Verification items for the finished model (mm, model axes). Coordinates: 2 decimals unless noted, no trailing zeros. Write each loop counter-clockwise with the first axis right and the second up, starting at its lowest first coordinate (ties: lowest second). Pieces come first, ordered by that corner, then holes. Notation, with made-up numbers: (33.5, -23.75) -> (60.5, -23.75) arc R11 ccw to (60.5, -5.75) -> close; hole circle Ø5 at (22.25, 17). An arc over 180 degrees is marked (long way). Answer in a Markdown table with one row per item.
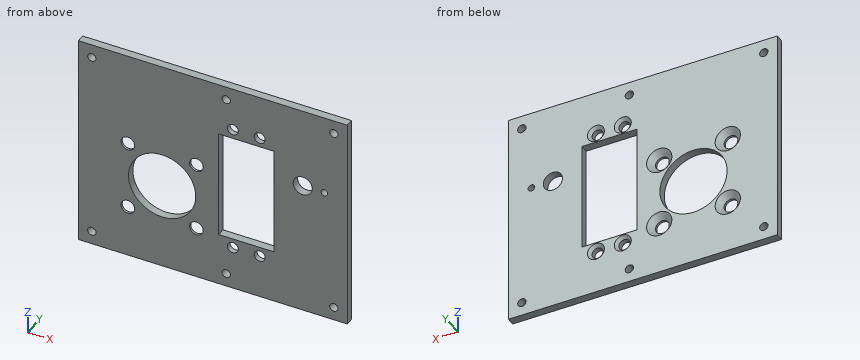
```python
from build123d import *

# Parameters (mm, degrees)
SZKIC1_W                                     = 100
SZKIC1_H                                     = 80
SZKIC1_R                                     = 12.5
SZKIC1_R_2                                   = 2.55
SZKIC1_R_3                                   = 2.05
SZKIC1_R_4                                   = 3.55
SZKIC1_R_5                                   = 1.55
SZKIC1_R_6                                   = 1.25
SZKIC1_W_2                                   = 20.5
SZKIC1_H_2                                   = 40.5
DODANIE_WYCI_GNI_CIE1_DEPTH                  = 3
CSK_FOR_M4_COUNTERSUNK_FLAT_HEAD_SCR_2_COUNT = 2
CSK_FOR_M4_COUNTERSUNK_FLAT_HEAD_SCR_2_PITCH = 25.5
CSK_FOR_M4_COUNTERSUNK_FLAT_HEAD_SCR_3_COUNT = 2
CSK_FOR_M4_COUNTERSUNK_FLAT_HEAD_SCR_3_PITCH = 36.062445841
CSK_FOR_M4_COUNTERSUNK_FLAT_HEAD_SCR_4_COUNT = 2
CSK_FOR_M4_COUNTERSUNK_FLAT_HEAD_SCR_4_PITCH = 25.5
CSK_FOR_M3_COUNTERSUNK_FLAT_HEAD_SCR_2_COUNT = 2
CSK_FOR_M3_COUNTERSUNK_FLAT_HEAD_SCR_2_PITCH = 10
CSK_FOR_M3_COUNTERSUNK_FLAT_HEAD_SCR_3_COUNT = 2
CSK_FOR_M3_COUNTERSUNK_FLAT_HEAD_SCR_3_PITCH = 47.5
CSK_FOR_M3_COUNTERSUNK_FLAT_HEAD_SCR_4_COUNT = 2
CSK_FOR_M3_COUNTERSUNK_FLAT_HEAD_SCR_4_PITCH = 48.541219597


with BuildPart() as part:
    # Szkic1 → Dodanie-wyciągnięcie1 (new body)
    with BuildSketch(Plane(origin=(0, 0, 0), x_dir=(1, 0, 0), z_dir=(0, 1, 0))):
        with Locations((11.336719097, -8.838965942)):
            Rectangle(SZKIC1_W, SZKIC1_H)
        with Locations((-7.518770099, -0.993104788)):
            Circle(SZKIC1_R, mode=Mode.SUBTRACT)
        with Locations((-20.268770099, 11.756895212)):
            Circle(SZKIC1_R_2, mode=Mode.SUBTRACT)
        with Locations((5.231229901, 11.756895212)):
            Circle(SZKIC1_R_2, mode=Mode.SUBTRACT)
        with Locations((5.231229901, -13.743104788)):
            Circle(SZKIC1_R_2, mode=Mode.SUBTRACT)
        with Locations((-20.268770099, -13.743104788)):
            Circle(SZKIC1_R_2, mode=Mode.SUBTRACT)
        with Locations((18.775116298, 14.911034058)):
            Circle(SZKIC1_R_3, mode=Mode.SUBTRACT)
        with Locations((28.775116298, 14.911034058)):
            Circle(SZKIC1_R_3, mode=Mode.SUBTRACT)
        with Locations((18.775116298, -32.588965942)):
            Circle(SZKIC1_R_3, mode=Mode.SUBTRACT)
        with Locations((28.775116298, -32.588965942)):
            Circle(SZKIC1_R_3, mode=Mode.SUBTRACT)
        with Locations((44.775116298, -18.788965942)):
            Circle(SZKIC1_R_4, mode=Mode.SUBTRACT)
        with Locations((-33.663280903, 26.161034058)):
            Circle(SZKIC1_R_5, mode=Mode.SUBTRACT)
        with Locations((56.336719097, 26.161034058)):
            Circle(SZKIC1_R_5, mode=Mode.SUBTRACT)
        with Locations((56.336719097, -43.838965942)):
            Circle(SZKIC1_R_5, mode=Mode.SUBTRACT)
        with Locations((-33.663280903, -43.838965942)):
            Circle(SZKIC1_R_5, mode=Mode.SUBTRACT)
        with Locations((16.336719097, 26.161034058)):
            Circle(SZKIC1_R_5, mode=Mode.SUBTRACT)
        with Locations((16.336719097, -43.838965942)):
            Circle(SZKIC1_R_5, mode=Mode.SUBTRACT)
        with Locations((52.775116298, -18.788965942)):
            Circle(SZKIC1_R_6, mode=Mode.SUBTRACT)
        with Locations((23.775116298, -8.838965942)):
            Rectangle(SZKIC1_W_2, SZKIC1_H_2, mode=Mode.SUBTRACT)
    extrude(amount=DODANIE_WYCI_GNI_CIE1_DEPTH)

    # Sketch4 → CSK for M4 Countersunk Flat Head Screw1 (revolve, cut)
    with BuildSketch(Plane(origin=(-20.268770099, 3, 13.743104788), x_dir=(0, 0, 1), z_dir=(1, 0, 0))):
        Polygon((0, 0), (0, 3), (2.25, 3), (2.25, 2.45), (4.7, 0), align=None)
    csk_for_m4_countersunk_flat_head_screw1 = revolve(axis=Axis((-20.268770099, 9.35, 13.743104788), (0, -1, 0)), mode=Mode.SUBTRACT)

    # CSK for M4 Countersunk Flat Head Scr 2: CSK for M4 Countersunk Flat Head Screw1 ×2
    with Locations(*[(i * CSK_FOR_M4_COUNTERSUNK_FLAT_HEAD_SCR_2_PITCH, 0, 0) for i in range(1, CSK_FOR_M4_COUNTERSUNK_FLAT_HEAD_SCR_2_COUNT)]):
        add(csk_for_m4_countersunk_flat_head_screw1, mode=Mode.SUBTRACT)

    # CSK for M4 Countersunk Flat Head Scr 3: CSK for M4 Countersunk Flat Head Screw1 ×2
    with Locations(*[Vector(0.707106781, 0, -0.707106781) * (i * CSK_FOR_M4_COUNTERSUNK_FLAT_HEAD_SCR_3_PITCH) for i in range(1, CSK_FOR_M4_COUNTERSUNK_FLAT_HEAD_SCR_3_COUNT)]):
        add(csk_for_m4_countersunk_flat_head_screw1, mode=Mode.SUBTRACT)

    # CSK for M4 Countersunk Flat Head Scr 4: CSK for M4 Countersunk Flat Head Screw1 ×2
    with Locations(*[(0, 0, -i * CSK_FOR_M4_COUNTERSUNK_FLAT_HEAD_SCR_4_PITCH) for i in range(1, CSK_FOR_M4_COUNTERSUNK_FLAT_HEAD_SCR_4_COUNT)]):
        add(csk_for_m4_countersunk_flat_head_screw1, mode=Mode.SUBTRACT)

    # Sketch6 → CSK for M3 Countersunk Flat Head Screw1 (revolve, cut)
    with BuildSketch(Plane(origin=(18.775116298, 3, -14.911034058), x_dir=(0, 0, 1), z_dir=(1, 0, 0))):
        Polygon((0, 0), (0, 3), (1.7, 3), (1.7, 1.45), (3.15, 0), align=None)
    csk_for_m3_countersunk_flat_head_screw1 = revolve(axis=Axis((18.775116298, 9.35, -14.911034058), (0, -1, 0)), mode=Mode.SUBTRACT)

    # CSK for M3 Countersunk Flat Head Scr 2: CSK for M3 Countersunk Flat Head Screw1 ×2
    with Locations(*[(i * CSK_FOR_M3_COUNTERSUNK_FLAT_HEAD_SCR_2_PITCH, 0, 0) for i in range(1, CSK_FOR_M3_COUNTERSUNK_FLAT_HEAD_SCR_2_COUNT)]):
        add(csk_for_m3_countersunk_flat_head_screw1, mode=Mode.SUBTRACT)

    # CSK for M3 Countersunk Flat Head Scr 3: CSK for M3 Countersunk Flat Head Screw1 ×2
    with Locations(*[(0, 0, i * CSK_FOR_M3_COUNTERSUNK_FLAT_HEAD_SCR_3_PITCH) for i in range(1, CSK_FOR_M3_COUNTERSUNK_FLAT_HEAD_SCR_3_COUNT)]):
        add(csk_for_m3_countersunk_flat_head_screw1, mode=Mode.SUBTRACT)

    # CSK for M3 Countersunk Flat Head Scr 4: CSK for M3 Countersunk Flat Head Screw1 ×2
    with Locations(*[Vector(0.206010481, 0, 0.978549785) * (i * CSK_FOR_M3_COUNTERSUNK_FLAT_HEAD_SCR_4_PITCH) for i in range(1, CSK_FOR_M3_COUNTERSUNK_FLAT_HEAD_SCR_4_COUNT)]):
        add(csk_for_m3_countersunk_flat_head_screw1, mode=Mode.SUBTRACT)


solid = part.part
```
1. Thickness scan on line 1 (X direction, y = 1.1, z = 32.5); line 2 (X direction, y = 2.9, z = 44); line 3 (X direction, y = 0.35, z = 14.5). Record the ranges inside material, lowest first. Write a range as from..to.
Geometry says:
| item | result |
|---|---|
| line 1 | -38.66..16.73, 20.82..26.73, 30.82..61.34 |
| line 2 | -38.66..-35.2, -32.12..14.8, 17.88..54.8, 57.88..61.34 |
| line 3 | -38.66..-22.7, -17.83..2.8, 7.67..13.53, 34.03..61.34 |
2. Section check A-A, the plane z = 26.5. Record the boundary of the cut face in (x, y), plus the area to 4 significant figures.
Geometry says:
| item | result |
|---|---|
| outline | (-38.66, 0) -> (13.53, 0) -> (13.53, 3) -> (-38.66, 3) -> close; (34.03, 0) -> (61.34, 0) -> (61.34, 3) -> (34.03, 3) -> close |
| area | 238.5 mm^2 |
3. Section check B-B, the plane x = -5. Record the boundary of the cut face in (y, z).
Geometry says:
| item | result |
|---|---|
| outline | (0, -31.16) -> (3, -31.16) -> (3, -11.25) -> (0, -11.25) -> close; (0, 13.24) -> (3, 13.24) -> (3, 48.84) -> (0, 48.84) -> close |
4. Section check C-C, the plane z = 2.5. Record the boundary of the cut face in (x, y), plus the area to 3 significant figures.
Geometry says:
| item | result |
|---|---|
| outline | (-38.66, 0) -> (-19.93, 0) -> (-19.93, 3) -> (-38.66, 3) -> close; (4.89, 0) -> (13.53, 0) -> (13.53, 3) -> (4.89, 3) -> close; (34.03, 0) -> (61.34, 0) -> (61.34, 3) -> (34.03, 3) -> close |
| area | 164 mm^2 |
